```python
from build123d import *

# Parameters (mm, degrees)
F1_DEPTH = 2.2098


with BuildPart() as f1:
    # F0 (on Top) → F1 (new body)
    with BuildSketch(Plane.XY):
        with BuildLine():
            Line((-49.268814, 54.850598), (-76.971687, 54.850598))
            Line((-76.971687, 54.850598), (-76.971687, 61.200598))
            Line((-76.971687, 61.200598), (-106.181687, 61.200598))
            Line((-106.181687, 61.200598), (-106.181687, 54.850598))
            Line((-106.181687, 54.850598), (-118.881687, 54.850598))
            Line((-118.881687, 54.850598), (-118.881687, 31.990598))
            Line((-118.881687, 31.990598), (-115.059145, 31.990598))
            Line((-115.059145, 31.990598), (-115.059145, 24.370598))
            ThreePointArc((-115.059145, 24.370598), (-111.711376, 16.288368), (-103.629145, 12.940598))
            Line((-103.629145, 12.940598), (-69.418213, 12.940598))
            ThreePointArc((-69.418213, 12.940598), (-65.203284, 8.306966), (-59.179145, 6.590598))
            Line((-59.179145, 6.590598), (-51.488371, 6.590598))
            ThreePointArc((-51.488371, 6.590598), (-48.648564, -2.299402), (-40.129145, -6.109402))
            Line((-40.129145, -6.109402), (-24.014959, -6.109402))
            ThreePointArc((-24.014959, -6.109402), (-20.028504, -17.370681), (-19.487546, -29.304481))
            Line((-19.487546, -29.304481), (22.481449, -29.304481))
            ThreePointArc((22.481449, -29.304481), (18.826755, 1.648605), (4.836249, 29.500285))
            ThreePointArc((4.836249, 29.500285), (10.191672, 39.231094), (20.218953, 44.008419))
            ThreePointArc((20.218953, 44.008419), (11.793317, 50.443192), (1.204081, 50.958689))
            Line((1.204081, 50.958689), (1.204081, 54.850598))
            Line((1.204081, 54.850598), (-13.695522, 54.850598))
            Line((-13.695522, 54.850598), (-19.180041, 63.403121))
            Line((-19.180041, 63.403121), (-43.784295, 63.403121))
            Line((-43.784295, 63.403121), (-49.268814, 54.850598))
        make_face()
        with BuildLine():
            Line((17.544895, -24.224481), (-14.205105, -24.224481))
            ThreePointArc((-14.205105, -24.224481), (-16.08053, -12.16415), (-21.079145, -1.029402))
            Line((-21.079145, -1.029402), (-40.129145, -1.029402))
            ThreePointArc((-40.129145, -1.029402), (-44.619273, 0.83047), (-46.479145, 5.320598))
            Line((-46.479145, 5.320598), (-46.479145, 11.670598))
            Line((-46.479145, 11.670598), (-59.179145, 11.670598))
            ThreePointArc((-59.179145, 11.670598), (-63.669273, 13.53047), (-65.529145, 18.020598))
            Line((-65.529145, 18.020598), (-103.629145, 18.020598))
            ThreePointArc((-103.629145, 18.020598), (-108.119273, 19.88047), (-109.979145, 24.370598))
            Line((-109.979145, 24.370598), (-109.979145, 37.070598))
            Line((-109.979145, 37.070598), (-113.801687, 37.070598))
            Line((-113.801687, 37.070598), (-113.801687, 49.770598))
            Line((-113.801687, 49.770598), (-101.101687, 49.770598))
            Line((-101.101687, 49.770598), (-101.101687, 56.120598))
            Line((-101.101687, 56.120598), (-82.051687, 56.120598))
            Line((-82.051687, 56.120598), (-82.051687, 49.770598))
            Line((-82.051687, 49.770598), (-46.491687, 49.770598))
            Line((-46.491687, 49.770598), (-41.007168, 58.323121))
            Line((-41.007168, 58.323121), (-21.957168, 58.323121))
            Line((-21.957168, 58.323121), (-16.472649, 49.770598))
            Line((-16.472649, 49.770598), (-3.875919, 49.770598))
            Line((-3.875919, 49.770598), (-3.875919, 42.150598))
            ThreePointArc((-3.875919, 42.150598), (2.608543, 46.074031), (10.174282, 45.625519))
            ThreePointArc((10.174282, 45.625519), (2.802737, 38.105), (-0.484488, 28.100399))
            ThreePointArc((-0.484488, 28.100399), (12.911162, 3.447489), (17.544895, -24.224481))
        make_face(mode=Mode.SUBTRACT)
    extrude(amount=F1_DEPTH)


solid = f1.part
```
The listing builds one solid part. Answer for the finished solid, in the listing's coordinates (mm). A direction names the side the tool comes from. Round coordinates to 2 decimals unless told otherwise and drop trailing zeros. Order: outer loops, then holes, each group sorted by start corner. A loop starts at its lowest first (then second) coordinate and runs counter-clockwise, first axis right, second up. Notation, with made-up numbers: (-19, 0.5) - (7, 0.5) arc R31 ccw to (7, 28.5) - close; hole circle Ø3 at (-0.5, -29). An arc over 180 degrees is marked (long way). Put each result on its own line as item: value. Start each with the question number.
(1) Given P1, Ø1.1, axis at x = -96, z = 0.5, coming from the -Y side; P2, Ø1.1, axis at x = -30, z = 0.5, coming from the -Y side; P3, Ø0.7, axis at y = 54, z = 1.5, coming from the +X side, each flat-ended and moving along its own axis, determine where each tip first touches the part or whether it passes through.
(2) Find section B-B (x = -85.5). Give the vertices of the cut face in (y, z).
(3) Find section A-A (y = 21.5). Give the vertices of the cut face in (x, z), plus the area to 3 significant figures.
(4) For faces 1 (the cylindrical face through (-65.279, 8.354, 1.089)), 2 (the cylindrical face through (10.077, 39.122, 1.089)), 3 (the flat face through (-43.788, 53.987, 1.089)), determine the directions among +Z, -Z, +X, -X, +Y, -Y from which every point of the face is accessible in a straight line to the end or side of a thin tool.
(5) Determine the mould class of faces 4 (the flat face through (-48, 10, 2.21)), 5 (the flat face through (-46.488, 59.187, 1.089)), 6 (the cylindrical face through (2.88, 38.23, 1.09)) for opening direction Y: released by +Y, released by -Y, zero draft, split by the parting line, or undercut.
(6) Straight lines are drawn through the part: probe 1 along Y at (x, z) = (-8.5, 1.6); probe 2 along Y at (x, z) = (-98, 1.95); probe 3 along Y at (x, z) = (11, 0.5). For each, find the intervals that lie inside material, in ascending order. Write a range as from..to.
Reply:
1. P1: y = 12.94
1. P2: y = -6.11
1. P3: x = 1.2
2. outline: (12.94, 0) - (18.02, 0) - (18.02, 2.21) - (12.94, 2.21) - close; (56.12, 0) - (61.2, 0) - (61.2, 2.21) - (56.12, 2.21) - close
3. outline: (-114.69, 0) - (-109.29, 0) - (-109.29, 2.21) - (-114.69, 2.21) - close; (4.19, 0) - (10.15, 0) - (10.15, 2.21) - (4.19, 2.21) - close
3. area: 25.1 mm^2
4. face 1: +Z, -Z, -X, -Y
4. face 2: +Z, -Z, +X
4. face 3: +Z, -Z
5. face 4: zero draft
5. face 5: released by +Y
5. face 6: undercut
6. probe 1: -29.3..-24.22, 49.77..54.85
6. probe 2: 12.94..18.02, 56.12..61.2
6. probe 3: -29.3..-24.22, 8.47..20.02, 39.95..50.71
